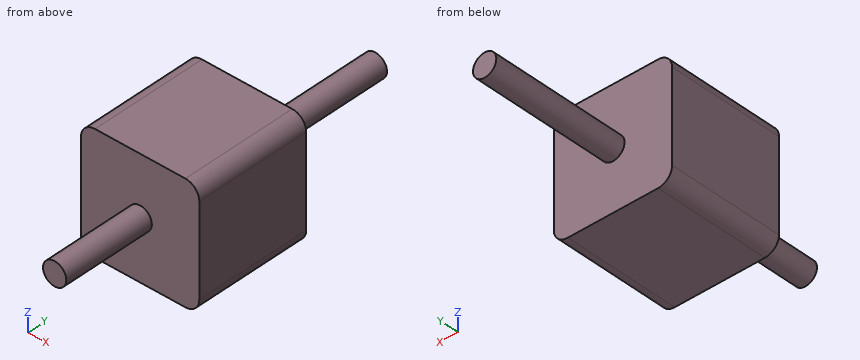
from build123d import *

# Parameters (mm, degrees)
BOSS_EXTRUDE1_DEPTH = 2.5
SKETCH2_R           = 0.25
BOSS_EXTRUDE2_DEPTH = 3
BOSS_EXTRUDE3_START = 2
SKETCH3_R           = 0.25
BOSS_EXTRUDE3_DEPTH = 2


with BuildPart() as part:
    # Sketch1 → Boss-Extrude1 (new body)
    with BuildSketch(Plane(origin=(0, 0, 0), x_dir=(1, 0, 0), z_dir=(0, 1, 0))):
        with BuildLine():
            Line((-0.97, -1.27), (0.97, -1.27))
            ThreePointArc((0.97, -1.27), (1.182132034, -1.182132034), (1.27, -0.97))
            Line((1.27, -0.97), (1.27, 0.97))
            ThreePointArc((1.27, 0.97), (1.182132034, 1.182132034), (0.97, 1.27))
            Line((0.97, 1.27), (-0.97, 1.27))
            ThreePointArc((-0.97, 1.27), (-1.182132034, 1.182132034), (-1.27, 0.97))
            Line((-1.27, 0.97), (-1.27, -0.97))
            ThreePointArc((-1.27, -0.97), (-1.182132034, -1.182132034), (-0.97, -1.27))
        make_face()
    extrude(amount=BOSS_EXTRUDE1_DEPTH)

    # Sketch2 → Boss-Extrude2 (add)
    with BuildSketch(Plane(origin=(0, 2.5, 0), x_dir=(1, 0, 0), z_dir=(0, 1, 0))):
        with Locations(Location((0, 0, 0), (0, 0, 270))):
            Circle(SKETCH2_R)
    extrude(amount=BOSS_EXTRUDE2_DEPTH)

    # Sketch3 → Boss-Extrude3 (add)
    with BuildSketch(Plane.XZ.offset(BOSS_EXTRUDE3_START)):
        with Locations(Location((0, 0, 0), (0, 0, 90))):
            Circle(SKETCH3_R)
    extrude(amount=-BOSS_EXTRUDE3_DEPTH)


solid = part.part
Work out the finished part from the listing and answer in its coordinate system (mm). Coordinates: 2 decimals unless noted, no trailing zeros. Loops run counter-clockwise (first coordinate to the right, second up) from the corner with the lowest first, then second, coordinate; pieces in that order, holes last. Notation, with made-up numbers: M 10,4.5 L 14,4.5 A21 ccw 14,25.5 Z; hole C 31,56 d10. An arc over 180 degrees is marked long. Answer in a Markdown table with one row per item. Add a question column.
1. Flat-ended cylindrical pins translate along their axes: P1, Ø0.8, axis at x = -0.5, z = 0.5, coming from the +Y side; P2, Ø1, axis at x = -0.5, y = 4.5, coming from the +Z side. Find the tip coordinate at first contact, or state that the pin passes through.
2. Consider L1, parallel to Y at x = 0.7, z = 0.6; L2, parallel to X at y = 1, z = -1; L3, parallel to X at y = 5.25, z = -0.1. Determine where each line is inside the solid, lowest interval first.
3. Find section A-A, the plane x = 0. Write down the section's boundary in (y, z).
4. Find section B-B, the plane z = 0.05. Write down the section's boundary in (x, y).
5. Find section C-C, the plane y = -1.5. Write down the section's boundary in (x, z).
6. Find section D-D, the plane x = -0.35. Write down the section's boundary in (y, z).
Reported:
| question | item | result |
|---|---|---|
| 1 | P1 | stops at y = 2.5 |
| 1 | P2 | stops at z = 0.25 |
| 2 | L1 | y = 0 to 2.5 |
| 2 | L2 | x = -1.27 to 1.27 |
| 2 | L3 | x = -0.23 to 0.23 |
| 3 | outline | M -2,-0.25 L 0,-0.25 L 0,-1.27 L 2.5,-1.27 L 2.5,-0.25 L 5.5,-0.25 L 5.5,0.25 L 2.5,0.25 L 2.5,1.27 L 0,1.27 L 0,0.25 L -2,0.25 Z |
| 4 | outline | M -1.27,0 L -0.24,0 L -0.24,-2 L 0.24,-2 L 0.24,0 L 1.27,0 L 1.27,2.5 L 0.24,2.5 L 0.24,5.5 L -0.24,5.5 L -0.24,2.5 L -1.27,2.5 Z |
| 5 | outline | C 0,0 d0.5 |
| 6 | outline | M 0,-1.27 L 2.5,-1.27 L 2.5,1.27 L 0,1.27 Z |
